from build123d import *

# Parameters (mm, degrees)
ESQUISSE1_W                   = 49.5
ESQUISSE1_H                   = 104.5
BOSS_EXTRU_1_DEPTH            = 139.8
COQUE1_T                      = -3
ENL_V_MAT_EXTRU_1_REACH       = 159.24
ESQUISSE2_W                   = 50
ESQUISSE2_H                   = 30
ESQUISSE3_W                   = 43.5
ESQUISSE3_H                   = 30
BOSS_EXTRU_2_DEPTH            = 2
ENL_V_MAT_EXTRU_2_REACH       = 153.283
ESQUISSE5_R                   = 10
ENL_V_MAT_EXTRU_3_REACH       = 150.516
ESQUISSE6_W                   = 43.5
ESQUISSE6_H                   = 41.5
ENL_V_MAT_EXTRU_4_REACH       = 153.283
ESQUISSE7_W                   = 6.9
ESQUISSE7_H                   = 12.7
D_PLACER_START                = 136.8
D_PLACER_LA_FACE1_OUTLINE_W   = 43.5
D_PLACER_LA_FACE1_OUTLINE_H   = 101.5
D_PLACER_LA_FACE1_OUTLINE_W_2 = 6.9
D_PLACER_LA_FACE1_OUTLINE_H_2 = 12.7
D_PLACER_LA_FACE1_OUTLINE_R   = 10
D_PLACER_LA_FACE1_DEPTH       = 0.2
D_PLACER_START_2              = 137
D_PLACER_LA_FACE1_2_DEPTH     = 2.8
ENL_V_MAT_EXTRU_5_REACH       = 176.525
ESQUISSE8_R                   = 1.2
D_PLACER_START_3              = 8.6
D_PLACER_LA_FACE2_OUTLINE_W   = 13.1
D_PLACER_LA_FACE2_OUTLINE_H   = 2.8
D_PLACER_LA_FACE2_DEPTH       = 7.3
BOSS_EXTRU_3_DEPTH            = 55
ESQUISSE10_R                  = 3.2
BOSS_EXTRU_4_DEPTH            = 2.5
ENL_V_MAT_EXTRU_6_DEPTH       = 152.283393008
ENL_V_MAT_EXTRU_6_DEPTH_BACK  = 1.22
ESQUISSE12_R                  = 4.05
ENL_V_MAT_EXTRU_7_REACH       = 175.083
ESQUISSE13_R                  = 1.2
ESQUISSE14_R                  = 2.5
ENL_V_MAT_EXTRU_8_DEPTH       = 3


# Read off the part's stored shape, not the designer's step: Déplacer la face1, Déplacer la face2
with BuildPart() as part:
    # Esquisse1 → Boss.-Extru.1 (new body)
    with BuildSketch(Plane.XY):
        Rectangle(ESQUISSE1_W, ESQUISSE1_H)
    extrude(amount=BOSS_EXTRU_1_DEPTH)

    # Coque1
    coque1_openings = [part.faces().sort_by_distance(p)[0] for p in [
        (0, 52.25, 69.9),
    ]]
    offset(amount=COQUE1_T, openings=coque1_openings, kind=Kind.INTERSECTION)

    # Esquisse2 → Enlèv. mat.-Extru.1 (cut, up to next)
    with BuildSketch(Plane(origin=(24.75, 0, 0), x_dir=(0, 0, -1), z_dir=(1, 0, 0)), mode=Mode.PRIVATE) as enl_v_mat_extru_1_sk1:
        with Locations((-25, 37.25)):
            Rectangle(ESQUISSE2_W, ESQUISSE2_H)
    enl_v_mat_extru_1_tool1 = extrude(enl_v_mat_extru_1_sk1.sketch, amount=-ENL_V_MAT_EXTRU_1_REACH, mode=Mode.PRIVATE) & part.part
    add(enl_v_mat_extru_1_tool1.solids().sort_by_distance((24.75, 37.25, 25))[0], mode=Mode.SUBTRACT)

    # Esquisse3 → Boss.-Extru.2 (add)
    with BuildSketch(Plane.XY.offset(3)):
        with Locations((0, -34.25)):
            Rectangle(ESQUISSE3_W, ESQUISSE3_H)
    extrude(amount=BOSS_EXTRU_2_DEPTH)

    # Esquisse5 → Enlèv. mat.-Extru.2 (cut, up to next)
    with BuildSketch(Plane.XY.offset(139.8), mode=Mode.PRIVATE) as enl_v_mat_extru_2_sk1:
        with Locations((0, 32.25)):
            Circle(ESQUISSE5_R)
    enl_v_mat_extru_2_tool1 = extrude(enl_v_mat_extru_2_sk1.sketch, amount=-ENL_V_MAT_EXTRU_2_REACH, mode=Mode.PRIVATE) & part.part
    add(enl_v_mat_extru_2_tool1.solids().sort_by_distance((0, 32.25, 139.8))[0], mode=Mode.SUBTRACT)

    # Esquisse6 → Enlèv. mat.-Extru.3 (cut, up to next)
    with BuildSketch(Plane.XY.offset(3), mode=Mode.PRIVATE) as enl_v_mat_extru_3_sk1:
        with Locations((0, 1.5)):
            Rectangle(ESQUISSE6_W, ESQUISSE6_H)
    enl_v_mat_extru_3_tool1 = extrude(enl_v_mat_extru_3_sk1.sketch, amount=-ENL_V_MAT_EXTRU_3_REACH, mode=Mode.PRIVATE) & part.part
    add(enl_v_mat_extru_3_tool1.solids().sort_by_distance((0, 1.5, 3))[0], mode=Mode.SUBTRACT)

    # Esquisse7 → Enlèv. mat.-Extru.4 (cut, up to next)
    with BuildSketch(Plane.XY.offset(139.8), mode=Mode.PRIVATE) as enl_v_mat_extru_4_sk1:
        Polygon((16.75, -47.15), (21.25, -47.15), (21.25, -48.75), (3.25, -48.75), (3.25, -47.15), (7.75, -47.15), (7.75, -43.99), (16.75, -43.99), align=None)
    enl_v_mat_extru_4_tool1 = extrude(enl_v_mat_extru_4_sk1.sketch, amount=-ENL_V_MAT_EXTRU_4_REACH, mode=Mode.PRIVATE) & part.part
    # Esquisse7 → Enlèv. mat.-Extru.4 (cut, up to next)
    with BuildSketch(Plane.XY.offset(139.8), mode=Mode.PRIVATE) as enl_v_mat_extru_4_sk2:
        with Locations((12.25, -33.99)):
            Rectangle(ESQUISSE7_W, ESQUISSE7_H)
    enl_v_mat_extru_4_tool2 = extrude(enl_v_mat_extru_4_sk2.sketch, amount=-ENL_V_MAT_EXTRU_4_REACH, mode=Mode.PRIVATE) & part.part
    add(enl_v_mat_extru_4_tool1.solids().sort_by_distance((12.25, -46.767484, 139.8))[0], mode=Mode.SUBTRACT)
    add(enl_v_mat_extru_4_tool2.solids().sort_by_distance((12.25, -33.99, 139.8))[0], mode=Mode.SUBTRACT)

    # Déplacer la face1 outline → Déplacer la face1 (cut)
    with BuildSketch(Plane.XY.offset(D_PLACER_START)):
        with Locations((0, 1.5)):
            Rectangle(D_PLACER_LA_FACE1_OUTLINE_W, D_PLACER_LA_FACE1_OUTLINE_H)
        Polygon((16.75, -43.99), (16.75, -47.15), (21.25, -47.15), (21.25, -48.75), (3.25, -48.75), (3.25, -47.15), (7.75, -47.15), (7.75, -43.99), align=None, mode=Mode.SUBTRACT)
        with Locations((12.25, -33.99)):
            Rectangle(D_PLACER_LA_FACE1_OUTLINE_W_2, D_PLACER_LA_FACE1_OUTLINE_H_2, mode=Mode.SUBTRACT)
        with Locations((0, 32.25)):
            Circle(D_PLACER_LA_FACE1_OUTLINE_R, mode=Mode.SUBTRACT)
    extrude(amount=D_PLACER_LA_FACE1_DEPTH, mode=Mode.SUBTRACT)

    # D_placer la face1 2 outline → D_placer la face1 2 (cut)
    with BuildSketch(Plane.XY.offset(D_PLACER_START_2)):
        Polygon((21.45, -46.95), (16.95, -46.95), (16.95, -43.79), (7.55, -43.79), (7.55, -46.95), (3.05, -46.95), (3.05, -48.95), (21.45, -48.95), align=None)
        Polygon((16.75, -43.99), (16.75, -47.15), (21.25, -47.15), (21.25, -48.75), (3.25, -48.75), (3.25, -47.15), (7.75, -47.15), (7.75, -43.99), align=None, mode=Mode.SUBTRACT)
    extrude(amount=D_PLACER_LA_FACE1_2_DEPTH, mode=Mode.SUBTRACT)

    # Esquisse8 → Enlèv. mat.-Extru.5 (cut, up to next)
    with BuildSketch(Plane(origin=(0, -49.25, 0), x_dir=(1, 0, 0), z_dir=(0, 1, 0)), mode=Mode.PRIVATE) as enl_v_mat_extru_5_sk1:
        with Locations(Location((19.25, -104.8, 0), (0, 0, 270))):
            Circle(ESQUISSE8_R)
    enl_v_mat_extru_5_tool1 = extrude(enl_v_mat_extru_5_sk1.sketch, amount=-ENL_V_MAT_EXTRU_5_REACH, mode=Mode.PRIVATE) & part.part
    # Esquisse8 → Enlèv. mat.-Extru.5 (cut, up to next)
    with BuildSketch(Plane(origin=(0, -49.25, 0), x_dir=(1, 0, 0), z_dir=(0, 1, 0)), mode=Mode.PRIVATE) as enl_v_mat_extru_5_sk2:
        with Locations(Location((5.25, -104.8, 0), (0, 0, 270))):
            Circle(ESQUISSE8_R)
    enl_v_mat_extru_5_tool2 = extrude(enl_v_mat_extru_5_sk2.sketch, amount=-ENL_V_MAT_EXTRU_5_REACH, mode=Mode.PRIVATE) & part.part
    add(enl_v_mat_extru_5_tool1.solids().sort_by_distance((19.25, -49.25, 104.8))[0], mode=Mode.SUBTRACT)
    add(enl_v_mat_extru_5_tool2.solids().sort_by_distance((5.25, -49.25, 104.8))[0], mode=Mode.SUBTRACT)

    # Déplacer la face2 outline → Déplacer la face2 (cut)
    with BuildSketch(Plane.YZ.offset(D_PLACER_START_3)):
        with Locations((-33.99, 138.4)):
            Rectangle(D_PLACER_LA_FACE2_OUTLINE_W, D_PLACER_LA_FACE2_OUTLINE_H)
    extrude(amount=D_PLACER_LA_FACE2_DEPTH, mode=Mode.SUBTRACT)

    # Esquisse9 → Boss.-Extru.3 (add)
    with BuildSketch(Plane(origin=(0, -49.25, 0), x_dir=(1, 0, 0), z_dir=(0, 1, 0))):
        Polygon((-0.25, -137), (-0.25, -77), (-21.75, -77), (-21.75, -75), (1.75, -75), (1.75, -137), align=None)
    extrude(amount=BOSS_EXTRU_3_DEPTH)

    # Esquisse10 → Boss.-Extru.4 (add)
    with BuildSketch(Plane(origin=(0, -49.25, 0), x_dir=(1, 0, 0), z_dir=(0, 1, 0))):
        with Locations(Location((14.000000445, -70.185602769, 0), (0, 0, 270))):
            Circle(ESQUISSE10_R)
        with Locations(Location((-13.999998962, -70.191367017, 0), (0, 0, 270))):
            Circle(ESQUISSE10_R)
        with Locations(Location((14.187545547, -9.685562878, 0), (0, 0, 270))):
            Circle(ESQUISSE10_R)
        with Locations(Location((-14.012453855, -9.691368299, 0), (0, 0, 270))):
            Circle(ESQUISSE10_R)
    extrude(amount=BOSS_EXTRU_4_DEPTH)

    # Esquisse12 → Enlèv. mat.-Extru.6 (cut, two sides: drawn at the far end of the back side and taken through both)
    with BuildSketch(Plane(origin=(0, 0, 0), x_dir=(-1, 0, 0), z_dir=(0, 0, -1)).offset(-ENL_V_MAT_EXTRU_6_DEPTH_BACK)):
        with Locations(Location((0, -27.5, 0), (0, 0, 180))):
            Circle(ESQUISSE12_R)
    extrude(amount=ENL_V_MAT_EXTRU_6_DEPTH + ENL_V_MAT_EXTRU_6_DEPTH_BACK, mode=Mode.SUBTRACT)

    # Esquisse13 → Enlèv. mat.-Extru.7 (cut, up to next)
    with BuildSketch(Plane(origin=(0, -46.75, 0), x_dir=(1, 0, 0), z_dir=(0, 1, 0)), mode=Mode.PRIVATE) as enl_v_mat_extru_7_sk1:
        with Locations(Location((14.187545547, -9.685562878, 0), (0, 0, 270))):
            Circle(ESQUISSE13_R)
    enl_v_mat_extru_7_tool1 = extrude(enl_v_mat_extru_7_sk1.sketch, amount=-ENL_V_MAT_EXTRU_7_REACH, mode=Mode.PRIVATE) & part.part
    # Esquisse13 → Enlèv. mat.-Extru.7 (cut, up to next)
    with BuildSketch(Plane(origin=(0, -46.75, 0), x_dir=(1, 0, 0), z_dir=(0, 1, 0)), mode=Mode.PRIVATE) as enl_v_mat_extru_7_sk2:
        with Locations(Location((-14.012453855, -9.691368299, 0), (0, 0, 270))):
            Circle(ESQUISSE13_R)
    enl_v_mat_extru_7_tool2 = extrude(enl_v_mat_extru_7_sk2.sketch, amount=-ENL_V_MAT_EXTRU_7_REACH, mode=Mode.PRIVATE) & part.part
    # Esquisse13 → Enlèv. mat.-Extru.7 (cut, up to next)
    with BuildSketch(Plane(origin=(0, -46.75, 0), x_dir=(1, 0, 0), z_dir=(0, 1, 0)), mode=Mode.PRIVATE) as enl_v_mat_extru_7_sk3:
        with Locations(Location((-13.999998962, -70.191367017, 0), (0, 0, 270))):
            Circle(ESQUISSE13_R)
    enl_v_mat_extru_7_tool3 = extrude(enl_v_mat_extru_7_sk3.sketch, amount=-ENL_V_MAT_EXTRU_7_REACH, mode=Mode.PRIVATE) & part.part
    # Esquisse13 → Enlèv. mat.-Extru.7 (cut, up to next)
    with BuildSketch(Plane(origin=(0, -46.75, 0), x_dir=(1, 0, 0), z_dir=(0, 1, 0)), mode=Mode.PRIVATE) as enl_v_mat_extru_7_sk4:
        with Locations(Location((14.000000445, -70.185602769, 0), (0, 0, 270))):
            Circle(ESQUISSE13_R)
    enl_v_mat_extru_7_tool4 = extrude(enl_v_mat_extru_7_sk4.sketch, amount=-ENL_V_MAT_EXTRU_7_REACH, mode=Mode.PRIVATE) & part.part
    add(enl_v_mat_extru_7_tool1.solids().sort_by_distance((14.187546, -46.75, 9.685563))[0], mode=Mode.SUBTRACT)
    add(enl_v_mat_extru_7_tool2.solids().sort_by_distance((-14.012454, -46.75, 9.691368))[0], mode=Mode.SUBTRACT)
    add(enl_v_mat_extru_7_tool3.solids().sort_by_distance((-13.999999, -46.75, 70.191367))[0], mode=Mode.SUBTRACT)
    add(enl_v_mat_extru_7_tool4.solids().sort_by_distance((14, -46.75, 70.185603))[0], mode=Mode.SUBTRACT)

    # Esquisse14 → Enlèv. mat.-Extru.8 (cut)
    with BuildSketch(Plane.XZ.offset(52.25)):
        with Locations(Location((14.187545547, 9.685562878, 0), (0, 0, 270))):
            Circle(ESQUISSE14_R)
        with Locations(Location((-14.012453855, 9.691368299, 0), (0, 0, 270))):
            Circle(ESQUISSE14_R)
        with Locations(Location((-13.999998962, 70.191367017, 0), (0, 0, 270))):
            Circle(ESQUISSE14_R)
        with Locations(Location((14.000000445, 70.185602769, 0), (0, 0, 270))):
            Circle(ESQUISSE14_R)
    extrude(amount=-ENL_V_MAT_EXTRU_8_DEPTH, mode=Mode.SUBTRACT)


solid = part.part
Design review of the part built by this model. Coordinates are the model's own, in mm. A direction names the side the tool comes from. Coordinates: 2 decimals unless noted, no trailing zeros. Loops run counter-clockwise (first coordinate to the right, second up) from the corner with the lowest first, then second, coordinate; pieces in that order, holes last. Notation, with made-up numbers: (13, 84) - (31, 84) arc R7 ccw to (31, 95) - close; hole circle Ø1 at (59.25, -0.75). An arc over 180 degrees is marked (long way). Use CSV: the item, a comma, the result in double quotes. Start each with the question number.
1. To check wall thickness, follow probe 1 along X at (y, z) = (-25, 86.5); probe 2 along X at (y, z) = (-50.5, 104.8); probe 3 along Z at (x, y) = (-4.5, -37.5). State the ranges of each line that lie inside material, in increasing order.
2. Add section C-C on y = 32.25. Give the boundary of the cut face in (x, z).
3. Add section A-A on y = -39. Give the boundary of the cut face in (x, z).
4. Add section B-B on z = 21.5. Give the boundary of the cut face in (x, y).
5. Mouldability with a two-part tool opening along Z and no side actions: class faces 6 (the flat face through (-6, -31, 0)), 7 (the flat face through (5, -46.95, 138)), 8 (the flat face through (-21.75, 1, 68)) as released by +Z, released by -Z, zero draft, split by the parting line, or undercut.
6. Clearance check with flat-ended pins moving along their axes: pin 1 (4 mm diameter, centred on x = -9.5, y = 41, fed in from -Z); pin 2 (6 mm diameter, centred on x = 14.19, z = 9.69, fed in from -Y); pin 3 (1.5 mm diameter, centred on x = -22.5, z = 29.5, fed in from +Y); pin 4 (1.5 mm diameter, centred on x = 13, z = 106, fed in from +Y). State where each tip first meets the part, or that it passes through.
7. For faces 1 (the cylindrical face through (-0.878, -23.546, 0.619)), 2 (the flat face through (16.95, -45, 138)), 3 (the flat face through (-10, -22, 75)), 4 (the flat face through (0, -19.25, 2)), 5 (the cylindrical face through (-15.5, -50.8, 11.7)), list the 3-axis set-ups (+Z, -Z, +X, -X, +Y, -Y) from which the entire face can be reached by the end or side of a thin tool; tool diameter is ignored.
8. Add section D-D on x = -8. Give the boundary of the cut face in (y, z).
Resolved:
1,probe 1,"-24.75 to -21.75, -0.25 to 1.75, 21.75 to 24.75"
1,probe 2,"-24.75 to 4.05, 6.45 to 18.05, 20.45 to 24.75"
1,probe 3,"0 to 5, 75 to 77, 137 to 139.8"
2,outline,"(-24.75, 50) - (-21.75, 50) - (-21.75, 137) - (-10, 137) - (-10, 139.8) - (-24.75, 139.8) - close; (10, 137) - (21.75, 137) - (21.75, 50) - (24.75, 50) - (24.75, 139.8) - (10, 139.8) - close"
3,outline,"(-24.75, 0) - (24.75, 0) - (24.75, 139.8) - (15.9, 139.8) - (15.9, 137) - (21.75, 137) - (21.75, 5) - (-21.75, 5) - (-21.75, 75) - (1.75, 75) - (1.75, 137) - (8.6, 137) - (8.6, 139.8) - (-24.75, 139.8) - close; hole (-21.75, 77) - (-0.25, 77) - (-0.25, 137) - (-21.75, 137) - close"
4,outline,"(-24.75, -52.25) - (24.75, -52.25) - (24.75, 22.25) - (21.75, 22.25) - (21.75, -49.25) - (-21.75, -49.25) - (-21.75, 22.25) - (-24.75, 22.25) - close"
5,face 6,"released by -Z"
5,face 7,"zero draft"
5,face 8,"undercut"
6,pin 1,"z = 137"
6,pin 2,"y = -52.25"
6,pin 3,"y = 22.25"
6,pin 4,"y = -49.25"
7,face 1,"-Z"
7,face 2,"+Z"
7,face 3,"+Y"
7,face 4,"-Z, +Y"
7,face 5,"-Y"
8,outline,"(-52.25, 0) - (-19.25, 0) - (-19.25, 5) - (-49.25, 5) - (-49.25, 75) - (5.75, 75) - (5.75, 77) - (-49.25, 77) - (-49.25, 137) - (26.25, 137) - (26.25, 139.8) - (-52.25, 139.8) - close; (38.25, 137) - (52.25, 137) - (52.25, 139.8) - (38.25, 139.8) - close"
